```python
from build123d import *

# Parameters (mm, degrees)
SM_BASE_FLANGE_1_DEPTH = 120
SKETCH_6_R             = 10
SKETCH_6_R_2           = 1.65
CUT_EXTRUDE_1_DEPTH    = 10
FILLET_1_R             = 3


# Sheet-metal steps are written as plain solids
with BuildPart() as part:
    # Sketch 1 → 基体-法兰1 (new body)
    with BuildSketch(Plane(origin=(0, 0, 0), x_dir=(1, 0, 0), z_dir=(0, 1, 0))):
        Polygon((0, 0), (-12, 0), (-12, 62), (102, 62), (102, 0), (90, 0), (90, -3), (105, -3), (105, 65), (-15, 65), (-15, -3), (0, -3), align=None)
    extrude(amount=-SM_BASE_FLANGE_1_DEPTH)

    # 草图6 → 切除-拉伸1 (cut)
    with BuildSketch(Plane(origin=(0, 0, -65), x_dir=(-1, 0, 0), z_dir=(0, 0, -1))):
        with Locations((-45, -60)):
            Circle(SKETCH_6_R)
        with Locations((-62.320508076, -70)):
            Circle(SKETCH_6_R_2)
        with Locations((-45, -40)):
            Circle(SKETCH_6_R_2)
        with Locations((-27.679491924, -70)):
            Circle(SKETCH_6_R_2)
    extrude(amount=-CUT_EXTRUDE_1_DEPTH, mode=Mode.SUBTRACT)

    # 圆角1
    fillet_1_edges = [part.edges().sort_by_distance(p)[0] for p in [
        (-15, -60, 3),
        (-15, -60, -65),
        (105, -60, -65),
        (105, -60, 3),
        (102, -60, 0),
        (102, -60, -62),
        (-12, -60, -62),
        (-12, -60, 0),
    ]]
    fillet(fillet_1_edges, radius=FILLET_1_R)


solid = part.part
```
The model under review builds one solid part; all positions refer to its coordinate system, in mm. A direction names the side the tool comes from. Give positions to 0.01 mm unless a question says otherwise; leave off trailing zeros. Order: outer loops, then holes, each group sorted by start corner. A loop starts at its lowest first (then second) coordinate and runs counter-clockwise, first axis right, second up. Notation, with made-up numbers: (75.25, 19.25) - (83.25, 19.25) arc R30 ccw to (83.25, 52.25) - close; hole circle Ø6 at (15.25, 39). An arc over 180 degrees is marked (long way). Use CSV: the item, a comma, the result in double quotes. Start each with the question number.
Q1. Clearance check with flat-ended pins moving along their axes: pin 1 Ø1.5 at (y, z) = (-38, 2) entering from -X; pin 2 Ø1.5 at (x, y) = (61, -85) entering from +Z; pin 3 Ø0.9 at (y, z) = (-82.5, 1) entering from +X. State where each tip first meets the part, or that it passes through.
Q2. We need section B-B, the plane z = -22. Write out the cut boundary in (x, y), and give its area (3 significant figures).
Q3. Tool access review of faces 1 (the cylindrical face through (101.1, -60.84, -61.14)), 2 (the cylindrical face through (53, -66, -64)): name each direction out of +Z, -Z, +X, -X, +Y, -Y from which nothing blocks a thin tool from reaching the whole face with its end or side.
Q4. We need section D-D, the plane y = -60. Write out the cut boundary in (x, z), and give its area (3 significant figures).
Q5. We need section C-C, the plane x = 45. Write out the cut boundary in (y, z), and give its area (3 significant figures).
Q6. The part is to be moulded in two halves that separate along Y. For faces 3 (the flat face through (45, -120, -64)), 4 (the cylindrical face through (46.216, -38.885, -63.521)), 5 (the flat face through (-4, -59, 0)), say which applies: +Y half, -Y half, draft (parallel to the pull), parting line (faces both ways), or undercut.
Q7. We need section A-A, the plane y = -40. Write out the cut boundary in (x, z), and give its area (3 significant figures).
Q8. To check wall thickness, follow line 1 along Y through (x, z) = (45, -63.9); line 2 along X through (y, z) = (-16, -30.5); line 3 along Z through (x, y) = (-1.5, -32.5). State the ranges of each line that lie inside material, in increasing order. Write a range as [from, to].
Outcome:
1,pin 1,"stops at x = -14.73"
1,pin 2,"stops at z = -62"
1,pin 3,"stops at x = 104.95"
2,outline,"(-15, -120) - (-12, -120) - (-12, 0) - (-15, 0) - close; (102, -120) - (105, -120) - (105, 0) - (102, 0) - close"
2,area,"720 mm^2"
3,face 1,"+Y, -Y"
3,face 2,"+Z, -Z"
4,outline,"(-15, -62) arc R3 ccw to (-12, -65) - (35, -65) - (35, -62) - (-9, -62) arc R3 cw to (-12, -59) - (-12, -3) arc R3 cw to (-9, 0) - (0, 0) - (0, 3) - (-12, 3) arc R3 ccw to (-15, 0) - close; (55, -65) - (102, -65) arc R3 ccw to (105, -62) - (105, 0) arc R3 ccw to (102, 3) - (90, 3) - (90, 0) - (99, 0) arc R3 cw to (102, -3) - (102, -59) arc R3 cw to (99, -62) - (55, -62) - close"
4,area,"762 mm^2"
5,outline,"(-120, -65) - (-70, -65) - (-70, -62) - (-120, -62) - close; (-50, -65) - (-41.65, -65) - (-41.65, -62) - (-50, -62) - close; (-38.35, -65) - (0, -65) - (0, -62) - (-38.35, -62) - close"
5,area,"290 mm^2"
6,face 3,"-Y half"
6,face 4,"undercut"
6,face 5,"draft"
7,outline,"(-15, -62) arc R3 ccw to (-12, -65) - (43.35, -65) - (43.35, -62) - (-9, -62) arc R3 cw to (-12, -59) - (-12, -3) arc R3 cw to (-9, 0) - (0, 0) - (0, 3) - (-12, 3) arc R3 ccw to (-15, 0) - close; (46.65, -65) - (102, -65) arc R3 ccw to (105, -62) - (105, 0) arc R3 ccw to (102, 3) - (90, 3) - (90, 0) - (99, 0) arc R3 cw to (102, -3) - (102, -59) arc R3 cw to (99, -62) - (46.65, -62) - close"
7,area,"812 mm^2"
8,line 1,"y = [-120, -70], [-50, -41.65], [-38.35, 0]"
8,line 2,"x = [-15, -12], [102, 105]"
8,line 3,"z = [-65, -62], [0, 3]"
